For this review, take the finished solid that the model builds, in its own axes (mm). A direction names the side the tool comes from. Give positions to 0.01 mm unless a question says otherwise; leave off trailing zeros. Order: outer loops, then holes, each group sorted by start corner. A loop starts at its lowest first (then second) coordinate and runs counter-clockwise, first axis right, second up. Notation, with made-up numbers: (17, 86.5) - (21, 86.5) arc R34 ccw to (21, 121.5) - close; hole circle Ø8 at (20, 8.5). An arc over 180 degrees is marked (long way). One line per item, written item: value.
```python
from build123d import *

# Parameters (mm, degrees)
F0_R     = 7.5
F1_DEPTH = 20
F2_SIZE2 = 7.1407400337
F2_SIZE  = 5
F3_R     = 5
F4_DEPTH = 3.2


with BuildPart() as f1:
    # F0 (on Top) → F1 (new body)
    with BuildSketch(Plane.XY):
        Circle(F0_R)
    extrude(amount=F1_DEPTH)

    # F2
    f2_edges = [f1.edges().sort_by_distance(p)[0] for p in [
        (-7.5, 0, 20),
    ]]
    f2_side = f1.faces().sort_by_distance((0, 0, 20))[0]
    chamfer(f2_edges, length=F2_SIZE, length2=F2_SIZE2, reference=f2_side)

    # F3 (on Top) → F4 (join)
    with BuildSketch(Plane.XY):
        Circle(F3_R)
    extrude(amount=-F4_DEPTH)


solid = f1.part
```
(1) Take a section at D-D (z = -0.5). Write out the cut boundary in (x, y).
Answers below:
outline: circle Ø10 at (0, 0)
(2) Take a section at C-C (z = 11). Write out the cut boundary in (x, y), then the cut area to 3 significant figures.
Answers below:
outline: circle Ø15 at (0, 0)
area: 177 mm^2
(3) For P1, Ø2, axis at x = -2.5, z = 0, coming from the -Y side; P2, Ø3, axis at x = -4.5, z = 3, coming from the +Y side, all flat-tipped, find the tip position at first contact; note any pin that passes through.
Answers below:
P1: stops at y = -7.35
P2: stops at y = 6.87
(4) Wall thickness on line 1 (Z direction, x = -1.5, y = -5.25); line 2 (X direction, y = 5.5, z = 4.25): over which ranges is each line inside the solid? List them lowest first. Write a range as from..to.
Answers below:
line 1: z = 0..15.77
line 2: x = -5.1..5.1
(5) Take a section at A-A (x = 0). Write out the cut boundary in (y, z).
Answers below:
outline: (-7.5, 0) - (-5, 0) - (-5, -3.2) - (5, -3.2) - (5, 0) - (7.5, 0) - (7.5, 12.86) - (2.5, 20) - (-2.5, 20) - (-7.5, 12.86) - close
(6) Machinability: for faces 1 (the face through (0, 0, 20)), 2 (the face through (2, -5, 0)), which of the approach directions +Z, -Z, +X, -X, +Y, -Y give a long, thin tool a straight path to every point of the face, cutting with its end or side? Answer none if there is none.
Answers below:
face 1: +Z, +X, -X, +Y, -Y
face 2: -Z
